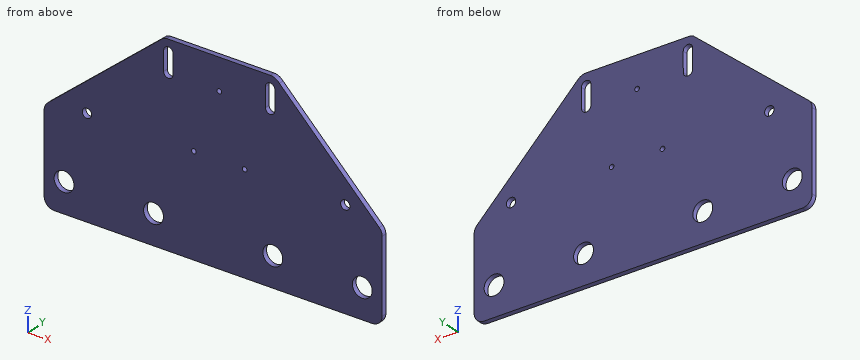
Autodesk Inventor part; units mm, degrees
ref_plane "YZ Plane" through (0, 0, 0) normal (1, 0, 0) x (0, 1, 0)
ref_plane "XZ Plane" through (0, 0, 0) normal (0, 1, 0) x (-1, 0, 0)
ref_plane "XY Plane" through (0, 0, 0) normal (0, 0, 1) x (1, 0, 0)
sketch "Sketch1" plane through (0, 0, 0) normal (0, 1, 0) x (-1, 0, 0)
  line L0 (-77.6185, -139.5068) -> (-293.5185, -139.5068)
  line L1 (-293.5185, -139.5068) -> (-293.5185, -291.9068)
  line L2 (-293.5185, -291.9068) -> (-77.6185, -291.9068)
  line L3 (-77.6185, -291.9068) -> (-77.6185, -139.5068)
  point P0 (0, 0)
  dimension "d0" = 215.9
  dimension "d1" = 152.4
extrude "Extrusion1" add sketch "Sketch1" along normal blind 3.175
sketch "Sketch2" plane through (0, 3.175, 0) normal (0, 1, 0) x (1, 0, 0)
  line L0 (77.6185, 291.9068) -> (77.6185, 139.5068)
  line L1 (77.6185, 139.5068) -> (293.5185, 139.5068)
  line L2 (293.5185, 139.5068) -> (293.5185, 291.9068)
  line L3 (293.5185, 291.9068) -> (77.6185, 291.9068)
  point P0 (0, 0)
  point P1 (156.9685, 165.5068)
  point P2 (104.9685, 218.5068)
  point P3 (269.9685, 218.5068)
  point P4 (221.9685, 165.5068)
  dimension "d4" = 144.35
  dimension "d5" = 26
  dimension "d7" = 79
  dimension "d19" = 27.35
  dimension "d20" = 79
  dimension "d21" = 26
  dimension "d22" = 79.35
  dimension "d23" = 192.35
hole "Hole1" at (156.9685, 3.175, -165.5068) at (104.9685, 3.175, -218.5068) at (269.9685, 3.175, -218.5068) at (221.9685, 3.175, -165.5068) direction (0, -1, 0) diameter 6 end through all
sketch "Sketch3" plane through (0, 3.175, 0) normal (0, 1, 0) x (1, 0, 0)
  line L0 (155.9994, 158.0068) -> (221.9685, 158.0068)
  circle A0 centre (221.9685, 165.5068) radius 3
  circle A1 centre (104.3905, 218.5068) radius 3
  circle A2 centre (156.9685, 165.5068) radius 3
  line L1 (153.2717, 158.9097) -> (79.8868, 220.4869)
  line L2 (77.6185, 139.5068) -> (293.5185, 139.5068)
  line L3 (293.5185, 229.1509) -> (293.5185, 276.0791)
  line L4 (293.5185, 291.9068) -> (77.6185, 291.9068)
  line L5 (77.6185, 291.9068) -> (77.6185, 139.5068)
  arc A3 (153.2717, 158.9097) -> (155.9994, 158.0068) centre (156.9685, 165.5068) ccw
  line L6 (96.6333, 206.4349) -> (77.6185, 222.3902)
  line L7 (48.2791, 233.5068) -> (391.5458, 233.5068) construction
  arc A4 (221.9685, 158.0068) -> (227.8466, 160.8487) centre (221.9685, 165.5068) ccw
  line L8 (227.8466, 160.8487) -> (291.6586, 224.6608)
  line L9 (293.5185, 226.5206) -> (293.5185, 282.4291)
  line L10 (293.5185, 139.5068) -> (293.5185, 291.9068)
  line L11 (287.1685, 282.4291) -> (83.9685, 282.4291)
  line L12 (77.6185, 276.0791) -> (77.6185, 225.3513)
  line L13 (77.6185, 291.9068) -> (77.6185, 139.5068)
  arc A5 (293.5185, 276.0791) -> (287.1685, 282.4291) centre (287.1685, 276.0791) ccw
  arc A6 (83.9685, 282.4291) -> (77.6185, 276.0791) centre (83.9685, 276.0791) ccw
  arc A7 (77.6185, 225.3513) -> (79.8868, 220.4869) centre (83.9685, 225.3513) ccw
  arc A8 (291.6586, 224.6608) -> (293.5185, 229.1509) centre (287.1685, 229.1509) ccw
  circle A9 centre (104.9685, 218.5068) radius 3
  line L14 (104.9685, 218.5068) -> (170.1885, 218.5068)
  point P0 (0, 0)
  point P1 (77.6185, 282.4291)
  point P2 (77.6185, 160.8487)
  dimension "d24" = 7.5
  dimension "d40" = 98.7582
  dimension "d72" = 6
  dimension "d93" = 7.5
  dimension "d96" = 52.578
  dimension "d99" = 135
  dimension "d100" = 6.35
  dimension "d101" = 6.35
  dimension "d102" = 6.35
  dimension "d103" = 6.35
  dimension "d104" = 140
  dimension "d127" = 9.4778
  dimension "d128" = 53
extrude "Extrusion3" cut sketch "Sketch3" against normal blind 25.4 contours L0 A4 L8 A8 L9 L10 L2 L5 L6 L1 A3 | L6 L5 A7 | A5 L11 A6 L5 L4 L10 L9
sketch "Sketch7" plane through (0, 3.175, 0) normal (0, 1, 0) x (1, 0, 0)
  circle A0 centre (156.9685, 165.5068) radius 3
  line L0 (155.9994, 158.0068) -> (221.9685, 158.0068)
  circle A1 centre (156.9685, 178.0036) radius 2.9972
  line L1 (153.9713, 178.0036) -> (153.9713, 165.3773)
  line L2 (159.9657, 178.0043) -> (159.9685, 165.5075)
  circle A2 centre (221.9713, 178.0036) radius 2.9972
  circle A3 centre (221.9685, 165.5068) radius 3
  line L3 (218.9741, 178.016) -> (218.9741, 165.3232)
  line L4 (224.9685, 178.0036) -> (224.9685, 165.5068)
  point P0 (0, 0)
  point P1 (218.9685, 165.5082)
  dimension "d76" = 5.9944
  dimension "d77" = 12.4968
  dimension "d78" = 5.9944
  dimension "d79" = 12.4968
  dimension "d88" = 6
extrude "Extrusion4" cut sketch "Sketch7" against normal blind 25.4 contours A0 L1 A1 L2 | A1
sketch "Sketch8" plane through (0, 3.175, 0) normal (0, 1, 0) x (1, 0, 0)
  arc A0 (224.9685, 178.0036) -> (218.9741, 177.9913) centre (221.9713, 178.0036) ccw
  circle A1 centre (221.9685, 165.5068) radius 3
  line L0 (218.9741, 178.016) -> (218.9741, 165.3232)
  line L1 (224.9685, 178.0036) -> (224.9685, 165.5068)
  point P0 (0, 0)
  point P1 (218.9685, 165.5082)
  dimension "d82" = 5.9944
  dimension "d83" = 12.4968
extrude "Extrusion5" cut sketch "Sketch8" against normal blind 25.4 contours L1 A1 L0 A0 | A1 L0 picked at (221.9464, 164.5591)
sketch "Sketch10" plane through (0, 3.175, 0) normal (0, 1, 0) x (1, 0, 0)
  line L0 (77.6185, 276.0791) -> (77.6185, 225.3513)
  line L1 (77.6185, 276.0791) -> (77.6185, 225.3513) construction
  line L2 (77.6185, 263.3791) -> (375.3248, 263.3791) construction
  line L3 (287.1685, 282.4291) -> (83.9685, 282.4291)
  line L4 (77.6185, 263.3791) -> (77.6185, 263.3791)
  point P0 (90.3185, 263.3791)
  point P1 (147.4685, 263.3791)
  point P2 (223.6685, 263.3791)
  point P3 (280.8185, 263.3791)
  dimension "d110" = 12.7
  dimension "d111" = 57.15
  dimension "d112" = 76.2
  dimension "d113" = 57.15
  dimension "d116" = 0.107
  dimension "d117" = 19.05
hole "Hole3" at (90.3185, 3.175, -263.3791) at (147.4685, 3.175, -263.3791) at (223.6685, 3.175, -263.3791) at (280.8185, 3.175, -263.3791) direction (0, -1, 0) diameter 12.7 depth 25.4 tip angle 118
sketch "Sketch5" plane through (0, 3.175, 0) normal (0, 1, 0) x (1, 0, 0)
  circle A0 centre (104.9685, 218.5068) radius 3
  circle A1 centre (104.9685, 218.5068) radius 22.225
  circle A2 centre (156.9685, 165.5068) radius 3
  circle A3 centre (156.9685, 165.5068) radius 22.225
  circle A4 centre (221.9685, 165.5068) radius 3
  circle A5 centre (221.9685, 165.5068) radius 22.225
  circle A6 centre (269.9685, 218.5068) radius 3
  circle A7 centre (269.9685, 218.5068) radius 22.225
  line L0 (155.9994, 158.0068) -> (221.9685, 158.0068)
  arc A8 (224.9685, 178.0036) -> (218.9741, 178.016) centre (221.9713, 178.0036) ccw
  line L1 (287.1685, 282.4291) -> (83.9685, 282.4291)
  point P0 (0, 0)
  point P1 (205.7185, 218.5096)
  point P2 (189.4685, 178.0036)
  point P3 (173.2185, 218.5096)
  dimension "d45" = 44.45
  dimension "d47" = 44.45
  dimension "d48" = 44.45
  dimension "d49" = 44.45
  dimension "d50" = 60.5028
  dimension "d52" = 65
  dimension "d53" = 16.25
  dimension "d54" = 16.25
  dimension "d55" = 60.5028
  dimension "d58" = 52
  dimension "d62" = 32.5
  dimension "d125" = 0
  dimension "d126" = 63.9194
hole "Hole2" at (205.7185, 3.175, -218.5096) at (189.4685, 3.175, -178.0036) at (173.2185, 3.175, -218.5096) direction (0, -1, 0) diameter 3 end through all
equation "\"d78\" = d76"
equation "\"d79\" = d77"
equation "\"d82\" = d84"
equation "\"d83\" = d85"
equation "\"d47\" = d45"
equation "\"d48\" = d45"
equation "\"d49\" = d48"
properties part number "track side panel V1"
For this review, take the finished solid that the model builds, in its own axes (mm). Give positions to 0.01 mm unless a question says otherwise; leave off trailing zeros. Order: outer loops, then holes, each group sorted by start corner. A loop starts at its lowest first (then second) coordinate and runs counter-clockwise, first axis right, second up.
1) Take a section at C-C (y = 0.9). State how many separate pieces and enclosed holes the cut face has, then the cut area to 3 significant figures.
2) Take a section at B-B (z = -174). Give the boundary of the cut face in (x, y) (1 decimal).
3) Insertion check: pin 1 (1 mm diameter, centred on y = 2, z = -172, fed in from -X); pin 2 (1.6 mm diameter, centred on y = 1.5, z = -172, fed in from +X); pin 3 (1.6 mm diameter, centred on y = 1.5, z = -169.5, fed in from -X). Each pin has a flat end and moves straight along its axis. Give the tip position at first contact, or say it passes through.
4) Wall thickness on line 1 (X direction, y = 2.2, z = -264); line 2 (X direction, y = 0.95, z = -262.5); line 3 (Z direction, x = 269, y = 0.15): over which ranges is each line inside the solid? List them lowest first.
5) Take a section at D-D (z = -210). Give the boundary of the cut face in (x, y) (3 decimals).
6) Take a section at A-A (x = 278). Give the boundary of the cut face in (y, z) (3 decimals).
Derived:
1. separate pieces: 1
1. enclosed holes: 11
1. area: 21,200 mm2
2. outline: (135.3, 0) - (154, 0) - (154, 3.2) - (135.3, 3.2) - close; (160, 0) - (219, 0) - (219, 3.2) - (160, 3.2) - close; (225, 0) - (241, 0) - (241, 3.2) - (225, 3.2) - close
3. pin 1: stops at x = 137.08
3. pin 2: stops at x = 239.8
3. pin 3: stops at x = 139.7
4. line 1: x = 77.62 to 84, 96.64 to 141.15, 153.79 to 217.35, 229.99 to 274.5, 287.14 to 293.52
4. line 2: x = 77.62 to 84.03, 96.61 to 141.18, 153.76 to 217.38, 229.96 to 274.53, 287.11 to 293.52
4. line 3: z = -282.43 to -221.35, -215.67 to -202
5. outline: (92.385, 0) - (276.998, 0) - (276.998, 3.175) - (92.385, 3.175) - close
6. outline: (0, -282.429) - (3.175, -282.429) - (3.175, -269.069) - (0, -269.069) - close; (0, -257.689) - (3.175, -257.689) - (3.175, -211.002) - (0, -211.002) - close
